Model file for the job. Use its own axes, mm. Round coordinates to 2 decimals unless told otherwise and drop trailing zeros. Order: outer loops, then holes, each group sorted by start corner. A loop starts at its lowest first (then second) coordinate and runs counter-clockwise, first axis right, second up. Notation, with made-up numbers: (63, 40) -> (112, 40) arc R15 cw to (112, 66) -> close; hole circle Ø11 at (-37, 15.25). An arc over 180 degrees is marked (long way). Put each result on its own line as item: value. Start each with the question number.
Q1. Probe L1, parallel to X at y = 0.7, z = 15; L2, parallel to X at y = 0.4, z = -15; L3, parallel to Z at x = 23, y = 0.6. List the from-to ranges inside material, lowest first.
Q2. Flat gauge pin, fed straight in: P1, Ø6, axis at x = -56.08, z = 0, coming from the -Y side. Where does the tip first touch, or does it go through?
Q3. Cut at D-D, the plane z = 30. List the corners of the cut face in (x, y).
Q4. Pull direction Z, two halves, no side cores. Call faces 1 (the face through (33.477, 0.493, 29.458)), 2 (the face through (-2, 0, -21)), 3 (the face through (-2.5, 0.5, 52.5)): released by +Z, released by -Z, zero draft, split by the parting line, or undercut.
Q5. Cut at A-A, the plane z = 15. List the corners of the cut face in (x, y), and give its area (3 significant figures).
Q6. Cut at C-C, the plane z = -10. List the corners of the cut face in (x, y), and give its area (3 significant figures).
Q7. Cut at B-B, the plane y = 0.65. State how many separate pieces and enclosed holes the cut face has, and give its area (3 significant figures).
from build123d import *

# Parameters (mm, degrees)
SKETCH1_R           = 35
SKETCH1_R_2         = 2.5
BOSS_EXTRUDE1_DEPTH = 1


with BuildPart() as part:
    # Sketch1 → Boss-Extrude1 (new body)
    with BuildSketch(Plane(origin=(0, 0, 0), x_dir=(1, 0, 0), z_dir=(0, 1, 0))):
        with BuildLine():
            Line((-66.082817056, 25), (-5.082817056, 25))
            ThreePointArc((-5.082817056, 25), (-2.582817056, 22.520776659), (-0.082817056, 25))
            Line((-0.082817056, 25), (60.917182944, 25))
            Line((60.917182944, 25), (60.917182944, -55))
            Line((60.917182944, -55), (-0.082817056, -55))
            ThreePointArc((-0.082817056, -55), (-2.582817056, -52.5), (-5.082817056, -55))
            Line((-5.082817056, -55), (-66.082817056, -55))
            Line((-66.082817056, -55), (-66.082817056, 25))
        make_face()
        with Locations(Location((-2.582817056, -15, 0), (0, 0, 270))):
            Circle(SKETCH1_R, mode=Mode.SUBTRACT)
        with Locations(Location((-56.082817056, 15, 0), (0, 0, 270))):
            Circle(SKETCH1_R_2, mode=Mode.SUBTRACT)
        with Locations(Location((-41.082817056, 15, 0), (0, 0, 270))):
            Circle(SKETCH1_R_2, mode=Mode.SUBTRACT)
        with Locations(Location((-56.082817056, 0, 0), (0, 0, 270))):
            Circle(SKETCH1_R_2, mode=Mode.SUBTRACT)
        with Locations(Location((-41.082817056, 0, 0), (0, 0, 270))):
            Circle(SKETCH1_R_2, mode=Mode.SUBTRACT)
        with Locations(Location((-26.082817056, 20.252893574, 0), (0, 0, 270))):
            Circle(SKETCH1_R_2, mode=Mode.SUBTRACT)
        with Locations(Location((-56.082817056, -15, 0), (0, 0, 270))):
            Circle(SKETCH1_R_2, mode=Mode.SUBTRACT)
        with Locations(Location((-41.082817056, -15, 0), (0, 0, 270))):
            Circle(SKETCH1_R_2, mode=Mode.SUBTRACT)
        with Locations(Location((50.917182944, 15, 0), (0, 0, 90))):
            Circle(SKETCH1_R_2, mode=Mode.SUBTRACT)
        with Locations(Location((50.917182944, 0, 0), (0, 0, 90))):
            Circle(SKETCH1_R_2, mode=Mode.SUBTRACT)
        with Locations(Location((50.917182944, -15, 0), (0, 0, 90))):
            Circle(SKETCH1_R_2, mode=Mode.SUBTRACT)
        with Locations(Location((35.917182944, -15, 0), (0, 0, 90))):
            Circle(SKETCH1_R_2, mode=Mode.SUBTRACT)
        with Locations(Location((35.917182944, 0, 0), (0, 0, 90))):
            Circle(SKETCH1_R_2, mode=Mode.SUBTRACT)
        with Locations(Location((35.917182944, 15, 0), (0, 0, 90))):
            Circle(SKETCH1_R_2, mode=Mode.SUBTRACT)
        with Locations(Location((20.917182944, 20.252893574, 0), (0, 0, 90))):
            Circle(SKETCH1_R_2, mode=Mode.SUBTRACT)
        with Locations(Location((-26.082817056, -50.252893574, 0), (0, 0, 90))):
            Circle(SKETCH1_R_2, mode=Mode.SUBTRACT)
        with Locations(Location((-41.082817056, -45, 0), (0, 0, 90))):
            Circle(SKETCH1_R_2, mode=Mode.SUBTRACT)
        with Locations(Location((-41.082817056, -30, 0), (0, 0, 90))):
            Circle(SKETCH1_R_2, mode=Mode.SUBTRACT)
        with Locations(Location((-56.082817056, -30, 0), (0, 0, 90))):
            Circle(SKETCH1_R_2, mode=Mode.SUBTRACT)
        with Locations(Location((-56.082817056, -45, 0), (0, 0, 90))):
            Circle(SKETCH1_R_2, mode=Mode.SUBTRACT)
        with Locations(Location((50.917182944, -45, 0), (0, 0, 270))):
            Circle(SKETCH1_R_2, mode=Mode.SUBTRACT)
        with Locations(Location((50.917182944, -30, 0), (0, 0, 270))):
            Circle(SKETCH1_R_2, mode=Mode.SUBTRACT)
        with Locations(Location((35.917182944, -30, 0), (0, 0, 270))):
            Circle(SKETCH1_R_2, mode=Mode.SUBTRACT)
        with Locations(Location((35.917182944, -45, 0), (0, 0, 270))):
            Circle(SKETCH1_R_2, mode=Mode.SUBTRACT)
        with Locations(Location((20.917182944, -50.252893574, 0), (0, 0, 270))):
            Circle(SKETCH1_R_2, mode=Mode.SUBTRACT)
    extrude(amount=BOSS_EXTRUDE1_DEPTH)


solid = part.part
Ans:
1. L1: x = -66.08 to -58.58, -53.58 to -43.58, -38.58 to -37.58, 32.42 to 33.42, 38.42 to 48.42, 53.42 to 60.92
1. L2: x = -66.08 to -58.58, -53.58 to -43.58, -38.58 to -20.61, 15.44 to 33.42, 38.42 to 48.42, 53.42 to 60.92
1. L3: z = -25 to -21.64, -18.87 to -8.89, 38.89 to 48.87, 51.64 to 55
2. P1: stops at y = 0
3. outline: (-66.08, 0) -> (-58.58, 0) -> (-58.58, 1) -> (-66.08, 1) -> close; (-53.58, 0) -> (-43.58, 0) -> (-43.58, 1) -> (-53.58, 1) -> close; (-38.58, 0) -> (-34.21, 0) -> (-34.21, 1) -> (-38.58, 1) -> close; (29.04, 0) -> (33.42, 0) -> (33.42, 1) -> (29.04, 1) -> close; (38.42, 0) -> (48.42, 0) -> (48.42, 1) -> (38.42, 1) -> close; (53.42, 0) -> (60.92, 0) -> (60.92, 1) -> (53.42, 1) -> close
4. face 1: undercut
4. face 2: zero draft
4. face 3: released by +Z
5. outline: (-66.08, 0) -> (-58.58, 0) -> (-58.58, 1) -> (-66.08, 1) -> close; (-53.58, 0) -> (-43.58, 0) -> (-43.58, 1) -> (-53.58, 1) -> close; (-38.58, 0) -> (-37.58, 0) -> (-37.58, 1) -> (-38.58, 1) -> close; (32.42, 0) -> (33.42, 0) -> (33.42, 1) -> (32.42, 1) -> close; (38.42, 0) -> (48.42, 0) -> (48.42, 1) -> (38.42, 1) -> close; (53.42, 0) -> (60.92, 0) -> (60.92, 1) -> (53.42, 1) -> close
5. area: 37.0 mm^2
6. outline: (-66.08, 0) -> (-27.08, 0) -> (-27.08, 1) -> (-66.08, 1) -> close; (21.91, 0) -> (60.92, 0) -> (60.92, 1) -> (21.91, 1) -> close
6. area: 78.0 mm^2
7. separate pieces: 1
7. enclosed holes: 25
7. area: 5,820 mm^2
